CAD build for the part. Positions are in the model's coordinates, mm. A direction names the side the tool comes from. Round coordinates to 2 decimals unless told otherwise and drop trailing zeros. Write each loop counter-clockwise with the first axis right and the second up, starting at its lowest first coordinate (ties: lowest second). Pieces come first, ordered by that corner, then holes. Notation, with made-up numbers: (2, 15) - (44, 15) arc R28 cw to (44, 48) - close; hole circle Ø10 at (71.25, -38). An arc over 180 degrees is marked (long way). Answer in a Markdown table with one row per item.
```python
from build123d import *

# Parameters (mm, degrees)
SKETCH1_W      = 34.0106
SKETCH1_H      = 29.9974
EXTRUDE1_DEPTH = 0.762
SKETCH2_W      = 27.9654
SKETCH2_H      = 27.9654
EXTRUDE2_DEPTH = 1.905
SKETCH3_W      = 29.9974
SKETCH3_H      = 29.9974
EXTRUDE3_DEPTH = 0.762
EXTRUDE4_START = 12.7
EXTRUDE4_DEPTH = 0.762


with BuildPart() as part:
    # Sketch1 → Extrude1 (new body)
    with BuildSketch(Plane(origin=(0, 0, 0), x_dir=(1, 0, 0), z_dir=(0, 1, 0))):
        Rectangle(SKETCH1_W, SKETCH1_H)
    extrude(amount=-EXTRUDE1_DEPTH)

    # Sketch2 → Extrude2 (add)
    with BuildSketch(Plane(origin=(0, 0, 0), x_dir=(-1, 0, 0), z_dir=(0, 1, 0))):
        with Locations((2.0066, 0)):
            Rectangle(SKETCH2_W, SKETCH2_H)
    extrude(amount=EXTRUDE2_DEPTH)

    # Sketch3 → Extrude3 (add)
    with BuildSketch(Plane(origin=(0, 1.905, 0), x_dir=(-1, 0, 0), z_dir=(0, 1, 0))):
        Rectangle(SKETCH3_W, SKETCH3_H)
    extrude(amount=EXTRUDE3_DEPTH)

    # Sketch4 → Extrude4 (add, symmetric)
    with BuildSketch(Plane.XY.offset(EXTRUDE4_START)):
        Polygon((13.8303, 0), (13.8303, 1.524), (20.1803, 1.524), (20.1803, 0.762), (17.0053, 0.762), (17.0053, 0), align=None)
    extrude4 = extrude(amount=EXTRUDE4_DEPTH, both=True)

    # Mirror1: Extrude4 across plane
    add(extrude4.mirror(Plane.XY))


solid = part.part
```
Q1. Flat gauge pins, fed straight in: pin 1 (1.5 mm diameter, centred on x = 14, y = 0.5, fed in from +Z); pin 2 (0.8 mm diameter, centred on x = -15.5, z = 5.5, fed in from +Y) (3 decimals); pin 3 (0.8 mm diameter, centred on x = 18, z = -12.5, fed in from -Y); pin 4 (1.2 mm diameter, centred on y = 1, z = 12.5, fed in from -X). Where does each tip first touch, or does it go through?
Computed:
| item | result |
|---|---|
| pin 1 | stops at z = 15 |
| pin 2 | stops at y = 1.905 |
| pin 3 | stops at y = 0.76 |
| pin 4 | stops at x = -15.99 |
Q2. Pull direction X, two halves, no side cores. Call faces 1 (the flat face through (13.83, 1, -13)), 2 (the flat face through (-15.989, 1, 0)), 3 (the flat face through (0, -0.762, 0)): released by +X, released by -X, zero draft, split by the parting line, or undercut.
Computed:
| item | result |
|---|---|
| face 1 | undercut |
| face 2 | released by -X |
| face 3 | zero draft |
Q3. Drill centre lines: line 1 (Y direction, x = 14, z = 5.75) (3 decimals); line 2 (X direction, y = 0.15, z = 10.5); line 3 (Z direction, x = -5, y = 0.6). Where is each one in solid material? Low to high.
Computed:
| item | result |
|---|---|
| line 1 | y = -0.762 to 0, 1.905 to 2.667 |
| line 2 | x = -15.99 to 11.98 |
| line 3 | z = -13.98 to 13.98 |
Q4. 3-axis set-ups, long thin cutter, end or side, ignore diameter. For faces 4 (the flat face through (-2, 1, -13.983)), 5 (the flat face through (13, 0, 0)), 6 (the flat face through (-2, 1, 13.983)), 7 (the flat face through (17.005, -0.3, 0.2)), 8 (the flat face through (17, 1.524, -13)): which of +Z, -Z, +X, -X, +Y, -Y reach the whole face in a straight line?
Computed:
| item | result |
|---|---|
| face 4 | -Z, +X, -X |
| face 5 | none |
| face 6 | +Z, +X, -X |
| face 7 | +Z, -Z, +X, -Y |
| face 8 | +Z, -Z, +X |
Q5. Saw through at B-B on x = 11. List the corners of the cut face in (y, z) (3 decimals), then the cut area to 3 significant figures.
Computed:
| item | result |
|---|---|
| outline | (-0.762, -14.999) - (0, -14.999) - (0, -13.983) - (1.905, -13.983) - (1.905, -14.999) - (2.667, -14.999) - (2.667, 14.999) - (1.905, 14.999) - (1.905, 13.983) - (0, 13.983) - (0, 14.999) - (-0.762, 14.999) - close |
| area | 99.0 mm2 |
Q6. Saw through at A-A on z = 13. List the corners of the cut face in (x, y) (3 decimals), then the cut area to 3 significant figures.
Computed:
| item | result |
|---|---|
| outline | (-17.005, -0.762) - (17.005, -0.762) - (17.005, 0.762) - (20.18, 0.762) - (20.18, 1.524) - (13.83, 1.524) - (13.83, 0) - (11.976, 0) - (11.976, 1.905) - (14.999, 1.905) - (14.999, 2.667) - (-14.999, 2.667) - (-14.999, 1.905) - (-15.989, 1.905) - (-15.989, 0) - (-17.005, 0) - close |
| area | 109 mm2 |
Q7. Saw through at C-C on z = 3. List the corners of the cut face in (x, y) (3 decimals).
Computed:
| item | result |
|---|---|
| outline | (-17.005, -0.762) - (17.005, -0.762) - (17.005, 0) - (11.976, 0) - (11.976, 1.905) - (14.999, 1.905) - (14.999, 2.667) - (-14.999, 2.667) - (-14.999, 1.905) - (-15.989, 1.905) - (-15.989, 0) - (-17.005, 0) - close |
